```python
from build123d import *
from OCP.BRepFilletAPI import BRepFilletAPI_MakeChamfer
from build123d.topology import SkipClean

# Parameters (mm, degrees)
SKETCH1_W                    = 6.604
SKETCH1_H                    = 11.43
BOSS_EXTRUDE1_DEPTH          = 74.93
SKETCH2_W                    = 14.6304
SKETCH2_H                    = 11.049
BOSS_EXTRUDE2_DEPTH          = 6.604
CUT_EXTRUDE1_DEPTH           = 79.507471982
SKETCH4_R                    = 3.175
CUT_EXTRUDE2_DEPTH           = 79.507471982
FILLET1_R                    = 4.7625
CHAMFER1_SIZE                = 3.175
CHAMFER1_SIZE2               = 1.833087105
CHAMFER2_SIZE                = 3.175
CHAMFER2_SIZE2               = 4.534369921
CHAMFER3_SIZE                = 3.81
CHAMFER3_SIZE2               = 4.540581188
BOSS_EXTRUDE3_DEPTH          = 3.048
F_1_8_0_125_DIAMETER_HOLE1_D = 3.175
FILLET2_R                    = 1.016


with BuildPart() as part:
    # Sketch1 → Boss-Extrude1 (new body)
    with BuildSketch(Plane.XY):
        with Locations((3.302, 5.715)):
            Rectangle(SKETCH1_W, SKETCH1_H)
    extrude(amount=BOSS_EXTRUDE1_DEPTH)

    # Sketch2 → Boss-Extrude2 (add)
    with BuildSketch(Plane(origin=(6.604, 0, 0), x_dir=(0, 0, -1), z_dir=(1, 0, 0))):
        with Locations((-7.3152, -5.5245)):
            Rectangle(SKETCH2_W, SKETCH2_H)
        with Locations((-7.3152, 16.9545)):
            Rectangle(SKETCH2_W, SKETCH2_H)
    extrude(amount=-BOSS_EXTRUDE2_DEPTH)

    # Sketch3 → Cut-Extrude1 (cut, through all)
    with BuildSketch(Plane(origin=(6.604, 0, 0), x_dir=(0, 0, -1), z_dir=(1, 0, 0))):
        Polygon((-10.922, 22.479), (-14.6304, 22.479), (-14.6304, 11.43), (-12.144086364, 11.43), align=None)
        Polygon((-14.6304, 0), (-14.6304, -11.049), (-13.408313636, 0), align=None)
    extrude(amount=-CUT_EXTRUDE1_DEPTH, mode=Mode.SUBTRACT)

    # Sketch4 → Cut-Extrude2 (cut, through all)
    with BuildSketch(Plane.XY.offset(74.93)):
        with Locations((8.1915, 5.715)):
            Circle(SKETCH4_R)
    extrude(amount=-CUT_EXTRUDE2_DEPTH, mode=Mode.SUBTRACT)

    # Fillet1
    fillet1_edges = [part.edges().sort_by_distance(p)[0] for p in [
        (0, -5.5245, 14.019356818),
        (0, 16.9545, 11.533043182),
    ]]
    fillet(fillet1_edges, radius=FILLET1_R)

    # Chamfer1
    chamfer1_edges = [part.edges().sort_by_distance(p)[0] for p in [
        (0, 5.715, 0),
    ]]
    chamfer1_side = [part.faces().sort_by_distance(p)[0] for p in [
        (0, 5.39199625, 31.764871667),
    ]]
    chamfer(chamfer1_edges, length=CHAMFER1_SIZE, length2=CHAMFER1_SIZE2, reference=chamfer1_side[0])

    # Chamfer2
    chamfer2_edges = [part.edges().sort_by_distance(p)[0] for p in [
        (6.604, 15.471815329, 0),
    ]]
    chamfer2_side = [part.faces().sort_by_distance(p)[0] for p in [
        (4.148704261, 5.715, 0),
    ]]
    chamfer(chamfer2_edges, length=CHAMFER2_SIZE, length2=CHAMFER2_SIZE2, reference=chamfer2_side[0])

    # Chamfer3: one chamfer whose edges measure the first distance from different faces: ONE call of the kernel's chamfer builder (chamfer() names one face for all edges)
    chamfer3_edges_1 = [part.edges().sort_by_distance(p)[0] for p in [
        (2.631043552, 22.479, 0),
    ]]
    chamfer3_side_1 = [part.faces().sort_by_distance(p)[0] for p in [
        (3.348233995, 22.479, 5.806565438),
    ]]
    chamfer3_edges_2 = [part.edges().sort_by_distance(p)[0] for p in [
        (2.631043552, -11.049, 0),
    ]]
    chamfer3_side_2 = [part.faces().sort_by_distance(p)[0] for p in [
        (2.631043552, 5.715, 0),
    ]]
    chamfer3 = BRepFilletAPI_MakeChamfer(part.part.solid().wrapped)
    for e in chamfer3_edges_1:
        chamfer3.Add(CHAMFER3_SIZE, CHAMFER3_SIZE2, e.wrapped, chamfer3_side_1[0].wrapped)  # the first distance lies on this face
    for e in chamfer3_edges_2:
        chamfer3.Add(CHAMFER3_SIZE, CHAMFER3_SIZE2, e.wrapped, chamfer3_side_2[0].wrapped)  # the first distance lies on this face
    add(Compound.cast(chamfer3.Shape()), mode=Mode.REPLACE)

    # Sketch5 → Boss-Extrude3 (add, symmetric)
    with BuildSketch(Plane(origin=(0, 5.715, 0), x_dir=(-1, 0, 0), z_dir=(0, -1, 0))):
        with BuildLine():
            Line((0, -74.93), (-6.604, -74.93))
            Line((-6.604, -74.93), (-7.921538097, -80.185366149))
            ThreePointArc((-7.921538097, -80.185366149), (-3.302, -86.106), (1.317538097, -80.185366149))
            Line((1.317538097, -80.185366149), (0, -74.93))
        make_face()
    extrude(amount=BOSS_EXTRUDE3_DEPTH, both=True)

    # 1/8 (0.125) Diameter Hole1 (through all)
    with Locations(Plane(origin=(0, 2.667, 0), x_dir=(-1, 0, 0), z_dir=(0, -1, 0))):
        with Locations((-3.302, -81.3435)):
            Hole(F_1_8_0_125_DIAMETER_HOLE1_D / 2)

    # Fillet2
    fillet2_edges = [part.edges().sort_by_distance(p)[0] for p in [
        (5.0165, 5.715, 74.93),
    ]]
    fillet(fillet2_edges, radius=FILLET2_R)

    # Sketch8 → Cut-Revolve3 (revolve, cut)
    with SkipClean():  # the faces are left unmerged after this step: merging them gives an invalid solid
        with BuildSketch(Plane(origin=(0, 5.715, 0), x_dir=(-1, 0, 0), z_dir=(0, -1, 0))):
            with BuildLine():
                ThreePointArc((-3.429, -44.7802), (-4.35893597, -42.53513597), (-6.604, -41.6052))
                Line((-6.604, -41.6052), (-6.604, -47.9552))
                ThreePointArc((-6.604, -47.9552), (-4.35893597, -47.02526403), (-3.429, -44.7802))
            make_face()
            with BuildLine():
                Line((-6.604, -47.9552), (-6.604, -41.6052))
                ThreePointArc((-6.604, -41.6052), (-9.779, -44.7802), (-6.604, -47.9552))
            make_face()
        revolve(axis=Axis((6.604, 5.715, 14.6304), (0, 0, 1)), mode=Mode.SUBTRACT)


solid = part.part
```
For this review, take the finished solid that the model builds, in its own axes (mm). A direction names the side the tool comes from. Coordinates: 2 decimals unless noted, no trailing zeros. Loops run counter-clockwise (first coordinate to the right, second up) from the corner with the lowest first, then second, coordinate; pieces in that order, holes last.
1. Add section C-C, the plane x = 0.75. Give the boundary of the cut face in (y, z).
2. Mouldability with a two-part tool opening along Z and no side actions: class faces 5 (the cylindrical face through (3, 5.8, 82.9)), 6 (the flat face through (2.614, -9.594, 2.807)), 7 (the cylindrical face through (1.43, -5.33, 12.63)), 8 (the flat face through (3, -11.049, 10)) as +Z half, -Z half, draft (parallel to the pull), parting line (faces both ways), or undercut.
3. Insertion check: P1, Ø0.8, axis at x = 5, y = 1, coming from the +Z side; P2, Ø2, axis at x = 1.5, z = 50, coming from the +Y side; P3, Ø0.6, axis at x = 6, y = 6, coming from the -Z side. Each pin has a flat end and moves straight along its axis. Give the tip position at first contact, or say it passes through.
4. For faces 1 (the cylindrical face through (5.017, 5.762, 22.745)), 2 (the flat face through (3, 10, 74.93)), 3 (the flat face through (3, 2.667, 79)), 4 (the flat face through (0, 6, 40)), list the 3-axis set-ups (+Z, -Z, +X, -X, +Y, -Y) from which the entire face can be reached by the end or side of a thin tool; tool diameter is ignored.
5. Add section B-B, the plane y = 1. Give the boundary of the cut face in (x, z) (3 decimals).
6. For line 1 (X direction, y = 9.5, z = 51.5); line 2 (Z direction, x = 2.5, y = 4); line 3 (Y direction, x = 6.5, z = 23.5), list the stretches that pass through material, from the lowest coordinate up.
Result:
1. outline: (-11.05, 4.54) - (-8.81, 1.88) - (20.17, 1.88) - (22.48, 3.81) - (22.48, 8.71) - (11.43, 9.93) - (11.43, 74.93) - (8.76, 74.93) - (8.76, 85.36) - (2.67, 85.36) - (2.67, 74.93) - (0, 74.93) - (0, 11.2) - (-11.05, 12.42) - close
2. face 5: undercut
2. face 6: -Z half
2. face 7: +Z half
2. face 8: draft
3. P1: stops at z = 74.93
3. P2: stops at y = 11.43
3. P3: stops at z = 74.87
4. face 1: -Z, +X
4. face 2: +Z, +X, -X, +Y
4. face 3: +Z, +X, -X, -Y
4. face 4: -Z, -X, +Y, -Y
5. outline: (0, 3.175) - (1.833, 0) - (3.429, 0) - (6.604, 4.534) - (6.604, 74.93) - (0, 74.93) - close
6. line 1: x = 0 to 6.6
6. line 2: z = 0 to 79.97, 82.71 to 86.04
6. line 3: y = 0 to 3.03, 8.4 to 11.43
